Here's the drawing with two shaded views (mm, measured from the low corner). I have some questions. Give positions to 0.01 mm unless a question says otherwise; leave off trailing zeros. Write each loop counter-clockwise with the first axis right and the second up, starting at its lowest first coordinate (ties: lowest second). Pieces come first, ordered by that corner, then holes. Notation, with made-up numbers: (14, 60.5) -> (21, 60.5) arc R12 ccw to (21, 72.5) -> close; hole circle Ø6 at (-7, 37). An arc over 180 degrees is marked (long way). One line per question, with ' | ' between items.
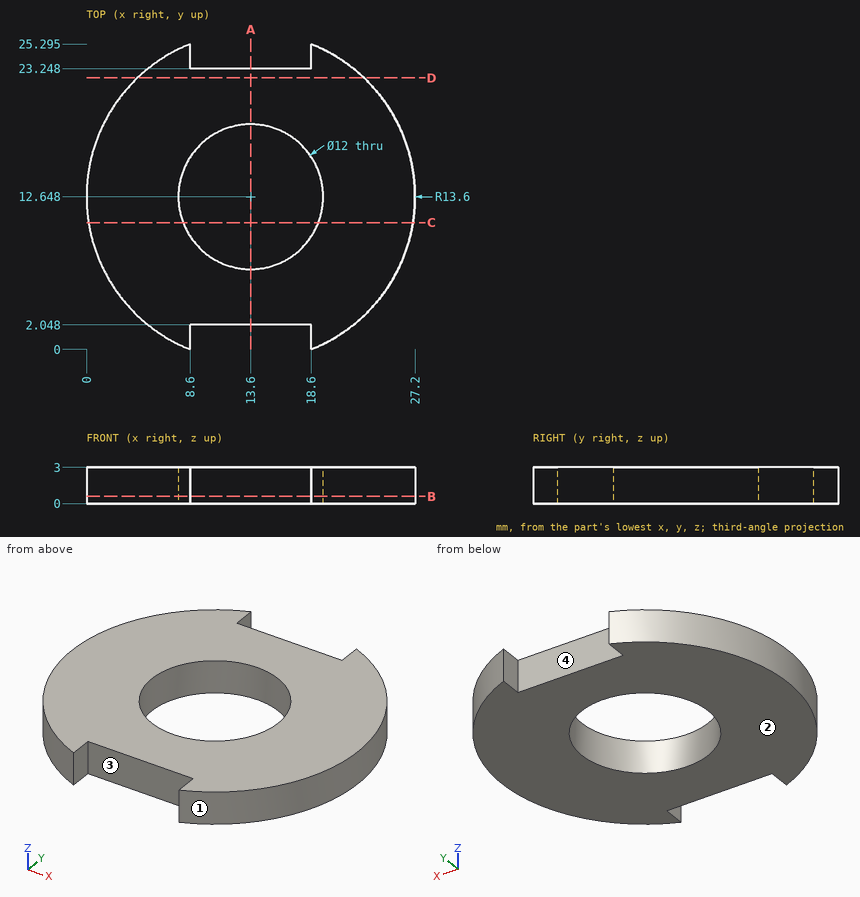
Q1. If I drill on line 1 along Y through (x, z) = (13.6, 2.05); line 2 along X through (y, z) = (1.5, 1.45); line 3 along X through (y, z) = (16.75, 1.3) (1 decimal), over which ranges is the centre line in solid material (lowest first)?
Answer below:
line 1: y = 2.05 to 6.65, 18.65 to 23.25 | line 2: x = 5.81 to 8.6, 18.6 to 21.39 | line 3: x = 0.6 to 9.2, 18 to 26.6
Q2. Imagine slicing it at C-C on y = 10.5. Please give me the cut outline in (x, z).
Answer below:
outline: (0.17, 0) -> (8, 0) -> (8, 3) -> (0.17, 3) -> close; (19.2, 0) -> (27.03, 0) -> (27.03, 3) -> (19.2, 3) -> close
Q3. Imagine slicing it at B-B on z = 0.6. Please give me the cut outline in (x, y) (1 decimal), and give its area (3 significant figures).
Answer below:
outline: (8.6, 0) -> (8.6, 2) -> (18.6, 2) -> (18.6, 0) arc R13.6 ccw to (18.6, 25.3) -> (18.6, 23.2) -> (8.6, 23.2) -> (8.6, 25.3) arc R13.6 ccw to start; hole circle Ø12 at (13.6, 12.6) | area: 414 mm^2
Q4. Will these pins go through, and if not, where does the flat tip stop? pin 1 (0.9 mm diameter, centred on x = 15.5, z = 1.5, fed in from +Y); pin 2 (0.6 mm diameter, centred on y = 1, z = 2, fed in from +X) (1 decimal); pin 3 (1 mm diameter, centred on y = 18.5, z = 1.5, fed in from +X).
Answer below:
pin 1: stops at y = 23.25 | pin 2: stops at x = 21.1 | pin 3: stops at x = 26.1
Q5. Imagine slicing it at D-D on y = 22.5. Please give me the cut outline in (x, z) (1 decimal).
Answer below:
outline: (4.2, 0) -> (23, 0) -> (23, 3) -> (4.2, 3) -> close
Q6. If we mould it in two halves opening along X, with no side actions, what happens to the marked faces 1, 2, 3 and 4? For each: +X half, -X half, draft (parallel to the pull), parting line (faces both ways), or undercut.
Answer below:
face 1: +X half | face 2: draft | face 3: undercut | face 4: undercut
Q7. Imagine slicing it at A-A on x = 13.6. Please give me the cut outline in (y, z), and give its area (3 significant figures).
Answer below:
outline: (2.05, 0) -> (6.65, 0) -> (6.65, 3) -> (2.05, 3) -> close; (18.65, 0) -> (23.25, 0) -> (23.25, 3) -> (18.65, 3) -> close | area: 27.6 mm^2
